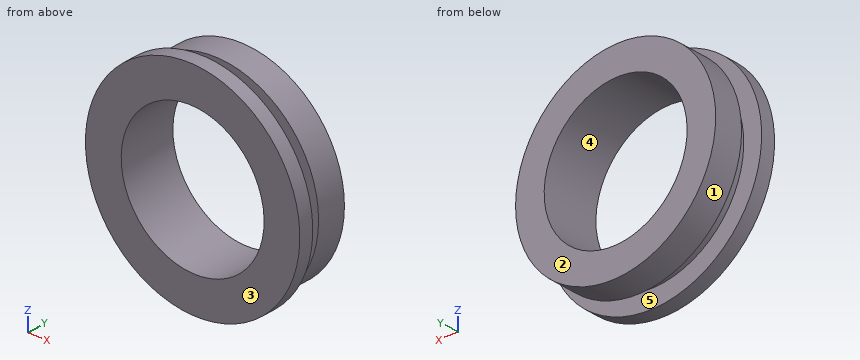
Autodesk Inventor part; units mm, degrees
ref_plane "YZ Plane" through (0, 0, 0) normal (1, 0, 0) x (0, 1, 0)
ref_plane "XZ Plane" through (0, 0, 0) normal (0, 1, 0) x (-1, 0, 0)
ref_plane "XY Plane" through (0, 0, 0) normal (0, 0, 1) x (1, 0, 0)
sketch "Sketch1" plane through (0, 0, 0) normal (1, 0, 0) x (0, 1, 0)
  line L0 (0, 0) -> (7.3009, 0)
  line L1 (0, -10) -> (8, -10)
  line L2 (0, -10) -> (0, -15)
  line L3 (0, -15) -> (2, -15)
  line L4 (2, -15) -> (2, -14)
  line L5 (2, -14) -> (8, -14)
  line L6 (8, -14) -> (8, -10)
  line L7 (2, -14) -> (2, -12.5)
  line L8 (2, -12.5) -> (4, -12.5)
  line L9 (4, -12.5) -> (4, -14)
  point P0 (4, -10)
  dimension "d0" = 20
  dimension "d1" = 6
  dimension "d2" = 2
  dimension "d3" = 28
  dimension "d4" = 30
  dimension "d8" = 2
  dimension "d9" = 1.5
revolve "Revolution1" add sketch "Sketch1" angle 360 about axis through (0, 0, 0) along (0, 1, 0) contours L1 L6 L5 L9 L8 L7 L4 L3 L2
thread "Thread1"
properties part number "034" material "Stainless Steel, Austenitic"
Could you check a few things on this model? Use its own coordinates, in mm. Face numbers are marked on the shaded views. A direction names the side the tool comes from. Coordinates: 2 decimals unless noted, no trailing zeros. Write each loop counter-clockwise with the first axis right and the second up, starting at its lowest first coordinate (ties: lowest second). Pieces come first, ordered by that corner, then holes. Notation, with made-up numbers: (67, -21.75) -> (112, -21.75) arc R12 ccw to (112, -8.75) -> close; hole circle Ø1 at (89, 78). An arc over 180 degrees is marked (long way). One line per question, with ' | ' between items. Start each with the question number.
1. Thinking about a two-plate mould opening in Y: for the marked faces 3, 4 and 5, which applies, pulls with the +Y half, pulls with the -Y half, needs draft (parallel to the pull), parting line crosses it, or undercut?
2. If we section it at D-D (z = 10.5): Please give me the cut outline in (x, y).
3. Please list where these lines run through material, in increasing order: line 1 along X through (y, z) = (6, 0); line 2 along Z through (x, y) = (0, 2.75).
4. For the marked faces 1 and 2, which set-ups out of +Z, -Z, +X, -X, +Y, -Y let a thin tool reach every point of the face, with its end or its side?
5. Will these pins go through, and if not, where does the flat tip stop? P1, Ø3, axis at x = 4.5, y = 5.5, coming from the +Z side; P2, Ø3, axis at y = 1.5, z = -10.5, coming from the +X side; P3, Ø3, axis at x = -5, y = 3, coming from the +Z side.
6. If we section it at C-C (y = 2.5): Please give me the cut outline in (x, z), and give its area (3 significant figures).
7. If we section it at B-B (z = 0): Please give me the cut outline in (x, y), and give its area (3 significant figures).
8. If we section it at A-A (x = 0): Please give me the cut outline in (y, z).
Return value:
1) face 3: pulls with the -Y half | face 4: needs draft | face 5: undercut
2) outline: (-10.71, 0) -> (10.71, 0) -> (10.71, 2) -> (6.78, 2) -> (6.78, 4) -> (9.26, 4) -> (9.26, 8) -> (-9.26, 8) -> (-9.26, 4) -> (-6.78, 4) -> (-6.78, 2) -> (-10.71, 2) -> close
3) line 1: x = -14 to -10, 10 to 14 | line 2: z = -12.5 to -10, 10 to 12.5
4) face 1: +Y | face 2: +Z, -Z, +X, -X, +Y
5) P1: stops at z = 13.67 | P2: stops at x = 12 | P3: stops at z = 14.49
6) outline: circle Ø25 at (0, 0); hole circle Ø20 at (0, 0) | area: 177 mm²
7) outline: (-15, 0) -> (-10, 0) -> (-10, 8) -> (-14, 8) -> (-14, 4) -> (-12.5, 4) -> (-12.5, 2) -> (-15, 2) -> close; (10, 0) -> (15, 0) -> (15, 2) -> (12.5, 2) -> (12.5, 4) -> (14, 4) -> (14, 8) -> (10, 8) -> close | area: 62.0 mm²
8) outline: (0, -15) -> (2, -15) -> (2, -12.5) -> (4, -12.5) -> (4, -14) -> (8, -14) -> (8, -10) -> (0, -10) -> close; (0, 10) -> (8, 10) -> (8, 14) -> (4, 14) -> (4, 12.5) -> (2, 12.5) -> (2, 15) -> (0, 15) -> close
